```python
from build123d import *

# Parameters (mm, degrees)
SKETCH1_W           = 50
SKETCH1_H           = 50
SKETCH1_R           = 15.2
SKETCH1_R_2         = 1.3
BOSS_EXTRUDE1_DEPTH = 30
CUT_EXTRUDE1_REACH  = 32
SKETCH2_W           = 3
SKETCH2_H           = 11.709133009
CUT_EXTRUDE2_DEPTH  = 54
CUT_EXTRUDE3_DEPTH  = 5


with BuildPart() as part:
    # Sketch1 → Boss-Extrude1 (new body)
    with BuildSketch(Plane.XY):
        with Locations((25, 25)):
            Rectangle(SKETCH1_W, SKETCH1_H)
        with Locations((25, 25)):
            Circle(SKETCH1_R, mode=Mode.SUBTRACT)
        with Locations((7, 15)):
            Circle(SKETCH1_R_2, mode=Mode.SUBTRACT)
        with Locations((7, 40)):
            Circle(SKETCH1_R_2, mode=Mode.SUBTRACT)
        with Locations((7, 10)):
            Circle(SKETCH1_R_2, mode=Mode.SUBTRACT)
        with Locations((7, 35)):
            Circle(SKETCH1_R_2, mode=Mode.SUBTRACT)
    extrude(amount=BOSS_EXTRUDE1_DEPTH)

    # Sketch2 → Cut-Extrude1 (cut, up to next)
    with BuildSketch(Plane.XY.offset(30), mode=Mode.PRIVATE) as cut_extrude1_sk1:
        with Locations((25, 5.854566505)):
            Rectangle(SKETCH2_W, SKETCH2_H)
    cut_extrude1_tool1 = extrude(cut_extrude1_sk1.sketch, amount=-CUT_EXTRUDE1_REACH, mode=Mode.PRIVATE) & part.part
    add(cut_extrude1_tool1.solids().sort_by_distance((25, 5.854567, 30))[0], mode=Mode.SUBTRACT)

    # Sketch3 → Cut-Extrude2 (cut)
    with BuildSketch(Plane(origin=(50, 0, 0), x_dir=(0, 0, -1), z_dir=(1, 0, 0))):
        Polygon((-11.940043573, 5), (-13.470021787, 7.65), (-16.529978213, 7.65), (-18.059956427, 5), (-16.529978213, 2.35), (-13.470021787, 2.35), align=None)
    extrude(amount=-CUT_EXTRUDE2_DEPTH, mode=Mode.SUBTRACT)

    # Sketch4 → Cut-Extrude3 (cut)
    with BuildSketch(Plane.ZY):
        Polygon((19.792007234, 5), (17.396003617, 9.15), (12.603996383, 9.15), (10.207992766, 5), (12.603996383, 0.85), (17.396003617, 0.85), align=None)
    extrude(amount=-CUT_EXTRUDE3_DEPTH, mode=Mode.SUBTRACT)


solid = part.part
```
The listing builds one solid part. Answer for the finished solid, in the listing's coordinates (mm). A direction names the side the tool comes from. Round coordinates to 2 decimals unless told otherwise and drop trailing zeros. Loops run counter-clockwise (first coordinate to the right, second up) from the corner with the lowest first, then second, coordinate; pieces in that order, holes last. Notation, with made-up numbers: (-19.5, 33) - (32.5, 33) arc R22 ccw to (32.5, 42) - close; hole circle Ø7 at (44.25, 82). An arc over 180 degrees is marked (long way). Return JSON: item names as keys, results as strings. Group by question number.
1. Consider probe 1 along Y at (x, z) = (7, 18.75); probe 2 along Y at (x, z) = (2, 13); probe 3 along Y at (x, z) = (7, 15.5). Determine where each line is inside the solid, lowest interval first.
2. The part is cut by section D-D on x = 13. Determine the outline of the cut face in (y, z).
3. The part is cut by section C-C on z = 25. Determine the outline of the cut face in (x, y).
4. The part is cut by section A-A on x = 7. Determine the outline of the cut face in (y, z), then the cut area to 3 significant figures.
5. The part is cut by section B-B on y = 25. Determine the outline of the cut face in (x, z), then the cut area to 3 significant figures.
6. Which of the six approach directions +Z, -Z, +X, -X, +Y, -Y give full straight-line access (tool end or side, diameter ignored) to faces 4 (the flat face through (26.5, 2, 15)), 5 (the flat face through (2.46, 2.9, 18.58)), 6 (the flat face through (14.38, 6.344, 17.284))?
7. The mould has two halves that part along Z. Classify faces 1 (the flat face through (14, 2.35, 15)), 2 (the flat face through (36, 36, 0)), 3 (the flat face through (50, 25, 15)): pulls with the +Z half, pulls with the -Z half, needs draft (parallel to the pull), parting line crosses it, or undercut.
Resolved:
{
 "1": {"probe 1": "y = 0 to 8.7, 11.3 to 13.7, 16.3 to 33.7, 36.3 to 38.7, 41.3 to 50", "probe 2": "y = 0 to 0.85, 9.15 to 50", "probe 3": "y = 0 to 2.35, 7.65 to 8.7, 11.3 to 13.7, 16.3 to 33.7, 36.3 to 38.7, 41.3 to 50"},
 "2": {"outline": "(0, 0) - (15.67, 0) - (15.67, 30) - (0, 30) - close; (34.33, 0) - (50, 0) - (50, 30) - (34.33, 30) - close; hole (2.35, 13.47) - (5, 11.94) - (7.65, 13.47) - (7.65, 16.53) - (5, 18.06) - (2.35, 16.53) - close"},
 "3": {"outline": "(0, 0) - (23.5, 0) - (23.5, 9.87) arc R15.2 cw (long way) to (26.5, 9.87) - (26.5, 0) - (50, 0) - (50, 50) - (0, 50) - close; hole circle Ø2.6 at (7, 10); hole circle Ø2.6 at (7, 15); hole circle Ø2.6 at (7, 35); hole circle Ø2.6 at (7, 40)"},
 "4": {"outline": "(0, 0) - (8.7, 0) - (8.7, 30) - (0, 30) - close; (11.3, 0) - (13.7, 0) - (13.7, 30) - (11.3, 30) - close; (16.3, 0) - (33.7, 0) - (33.7, 30) - (16.3, 30) - close; (36.3, 0) - (38.7, 0) - (38.7, 30) - (36.3, 30) - close; (41.3, 0) - (50, 0) - (50, 30) - (41.3, 30) - close; hole (2.35, 13.47) - (5, 11.94) - (7.65, 13.47) - (7.65, 16.53) - (5, 18.06) - (2.35, 16.53) - close", "area": "1,160 mm²"},
 "5": {"outline": "(0, 0) - (9.8, 0) - (9.8, 30) - (0, 30) - close; (40.2, 0) - (50, 0) - (50, 30) - (40.2, 30) - close", "area": "588 mm²"},
 "6": {"face 4": "+Z, -Z, -Y", "face 5": "-X", "face 6": "+X, -X"},
 "7": {"face 1": "undercut", "face 2": "pulls with the -Z half", "face 3": "needs draft"}
}
